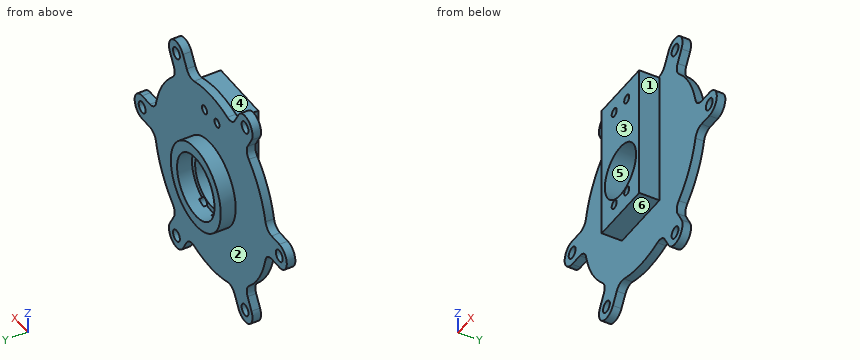
```python
from build123d import *

# Parameters (mm, degrees)
SKETCH_1_R               = 20
SKETCH_1_R_2             = 15
EXTRUDE_1_DEPTH          = 7
SKETCH_2_R               = 70
SKETCH_2_R_2             = 12.5
EXTRUDE_2_DEPTH          = 4
SKETCH_3_W               = 30
SKETCH_3_H               = 64
SKETCH_3_R               = 2
SKETCH_3_R_2             = 12.5
EXTRUDE_3_DEPTH          = 9.5
SKETCH_4_R               = 80
SKETCH_4_R_2             = 45
CUT_EXTRUDE_1_DEPTH      = 9.5
CUT_EXTRUDE_START        = -15
SKETCH_6_R               = 2
CUT_EXTRUDE_2_DEPTH      = 15
SKETCH_7_R               = 2.75
EXTRUDE_4_DEPTH          = 4
PATTERN_CIRCULAR_1_COUNT = 6
FILLET_2_R               = 5


with BuildPart() as part:
    # Эскиз1 → Бобышка-Вытянуть1 (new body)
    with BuildSketch(Plane(origin=(0, 0, 0), x_dir=(1, 0, 0), z_dir=(0, 1, 0))):
        with Locations(Location((0, 0, 0), (0, 0, 270))):
            Circle(SKETCH_1_R)
        with Locations(Location((0, 0, 0), (0, 0, 270))):
            Circle(SKETCH_1_R_2, mode=Mode.SUBTRACT)
    extrude(amount=EXTRUDE_1_DEPTH)

    # Эскиз2 → Бобышка-Вытянуть2 (add)
    with BuildSketch(Plane.XZ):
        with Locations(Location((0, 0, 0), (0, 0, 270))):
            Circle(SKETCH_2_R)
        with Locations(Location((0, 0, 0), (0, 0, 270))):
            Circle(SKETCH_2_R_2, mode=Mode.SUBTRACT)
    extrude(amount=EXTRUDE_2_DEPTH)

    # Эскиз3 → Бобышка-Вытянуть3 (add)
    with BuildSketch(Plane.XZ.offset(4)):
        with Locations((0, 10)):
            Rectangle(SKETCH_3_W, SKETCH_3_H)
        with Locations(Location((-5, 34, 0), (0, 0, 270))):
            Circle(SKETCH_3_R, mode=Mode.SUBTRACT)
        with Locations(Location((5, 34, 0), (0, 0, 270))):
            Circle(SKETCH_3_R, mode=Mode.SUBTRACT)
        with Locations(Location((-5, -14, 0), (0, 0, 270))):
            Circle(SKETCH_3_R, mode=Mode.SUBTRACT)
        with Locations(Location((5, -14, 0), (0, 0, 270))):
            Circle(SKETCH_3_R, mode=Mode.SUBTRACT)
        with Locations(Location((0, 0, 0), (0, 0, 270))):
            Circle(SKETCH_3_R_2, mode=Mode.SUBTRACT)
    extrude(amount=EXTRUDE_3_DEPTH)

    # Эскиз4 → Вырез-Вытянуть1 (cut)
    with BuildSketch(Plane(origin=(0, 0, 0), x_dir=(1, 0, 0), z_dir=(0, 1, 0))):
        Circle(SKETCH_4_R)
        with Locations(Location((0, 0, 0), (0, 0, 270))):
            Circle(SKETCH_4_R_2, mode=Mode.SUBTRACT)
    extrude(amount=-CUT_EXTRUDE_1_DEPTH, mode=Mode.SUBTRACT)

    # Эскиз6 → Вырез-Вытянуть2 (cut)
    with BuildSketch(Plane.XZ.offset(13.5).offset(CUT_EXTRUDE_START)):
        with Locations(Location((-5, 34, 0), (0, 0, 270))):
            Circle(SKETCH_6_R)
        with Locations(Location((5, 34, 0), (0, 0, 270))):
            Circle(SKETCH_6_R)
        with Locations(Location((-5, -14, 0), (0, 0, 160.346175942))):
            Circle(SKETCH_6_R)
        with Locations(Location((5, -14, 0), (0, 0, 19.653824058))):
            Circle(SKETCH_6_R)
    extrude(amount=CUT_EXTRUDE_2_DEPTH, mode=Mode.SUBTRACT)

    # Эскиз7 → Бобышка-Вытянуть4 (add)
    with BuildSketch(Plane(origin=(0, 0, 0), x_dir=(1, 0, 0), z_dir=(0, 1, 0))):
        with BuildLine():
            Line((-55, 6), (-40, 6))
            Line((-40, 6), (-40, -6))
            Line((-40, -6), (-55, -6))
            ThreePointArc((-55, -6), (-61, 0), (-55, 6))
        make_face()
        with Locations(Location((-55, 0, 0), (0, 0, 270))):
            Circle(SKETCH_7_R, mode=Mode.SUBTRACT)
    extrude_4 = extrude(amount=-EXTRUDE_4_DEPTH)

    # Круговой массив1: Бобышка-Вытянуть4 ×6 about axis
    pattern_circular_1_axis = Axis((0, 0, 0), (0, 1, 0))
    for i in range(1, PATTERN_CIRCULAR_1_COUNT):
        add(extrude_4.rotate(pattern_circular_1_axis, i * 360 / PATTERN_CIRCULAR_1_COUNT))

    # Скругление2
    fillet_2_edges = [part.edges().sort_by_distance(p)[0] for p in [
        (-17.102950698, -2, 41.623179569),
        (-27.495255544, -2, 35.623179569),
        (27.495255544, -2, 35.623179569),
        (17.102950698, -2, 41.623179569),
        (44.598206242, -2, -6),
        (44.598206242, -2, 6),
        (17.102950698, -2, -41.623179569),
        (27.495255544, -2, -35.623179569),
        (-27.495255544, -2, -35.623179569),
        (-17.102950698, -2, -41.623179569),
        (-44.598206242, -2, 6),
        (-44.598206242, -2, -6),
    ]]
    fillet(fillet_2_edges, radius=FILLET_2_R)


solid = part.part
```
Verification items for the finished model (mm, model axes). Face numbers are marked on the shaded views. A direction names the side the tool comes from. Give positions to 0.01 mm unless a question says otherwise; leave off trailing zeros. Order: outer loops, then holes, each group sorted by start corner. A loop starts at its lowest first (then second) coordinate and runs counter-clockwise, first axis right, second up. Notation, with made-up numbers: M 80.5,-39 L 132.5,-39 A29 ccw 132.5,-17 Z; hole C 47.5,-36.5 d11. An arc over 180 degrees is marked long. Return JSON: item names as keys, results as strings. Group by question number.
1) Mould release check, pull along Z, two halves, no side actions. Record for the marked faces 3, 4, 5 and 6: pulls with the +Z half, pulls with the -Z half, needs draft (parallel to the pull), parting line crosses it, or undercut.
2) Access from +Z, -Z, +X, -X, +Y, -Y to the whole of each face (thin tool, end or side, straight path). Record for the marked faces 1 and 2.
3) Section check B-B on x = -27.5. Record the cut outline in (y, z), and give its area (3 significant figures).
4) Section check C-C on y = -11.25. Record the cut outline in (x, z), and give its area (3 significant figures).
5) Scan lines: line 1 (X direction, y = -2.75, z = 0); line 2 (X direction, y = -1.5, z = -1); line 3 (Y direction, x = 43, z = 2). Record each from-to range of solid material in increasing order.
6) Section check D-D on x = 0. Record the cut outline in (y, z).
7) Section check A-A on z = 0. Record the cut outline in (x, y).
8) Go/stop test with flat-tipped pins: pin 1 Ø8 at (x, y) = (-23, 1.5) entering from +Z; pin 2 Ø10.5 at (y, z) = (-9.5, 2) entering from +X; pin 3 Ø2 at (x, y) = (51, -2.5) entering from +Z; pin 4 Ø3.5 at (x, z) = (5, 34) entering from +Y. Record where each tip stops, or that it passes through.
Answer block:
{
 "1": {"face 3": "needs draft", "face 4": "pulls with the +Z half", "face 5": "undercut", "face 6": "pulls with the -Z half"},
 "2": {"face 1": "+Z, -Z, +X, -Y", "face 2": "+Y"},
 "3": {"outline": "M -4,-53.63 L 0,-53.63 L 0,-50.38 L -4,-50.38 Z; M -4,-44.88 L 0,-44.88 L 0,44.88 L -4,44.88 Z; M -4,50.38 L 0,50.38 L 0,53.63 L -4,53.63 Z", "area": "385 mm^2"},
 "4": {"outline": "M -15,-22 L 15,-22 L 15,42 L -15,42 Z; hole C 0,0 d25; hole C -5,-14 d4; hole C -5,34 d4; hole C 5,-14 d4; hole C 5,34 d4", "area": "1,380 mm^2"},
 "5": {"line 1": "x = -61 to -57.75, -52.25 to -12.5, 12.5 to 52.25, 57.75 to 61", "line 2": "x = -60.92 to -57.56, -52.44 to -12.46, 12.46 to 52.44, 57.56 to 60.92", "line 3": "y = -4 to 0"},
 "6": {"outline": "M -13.5,-22 L -4,-22 L -4,-45 L 0,-45 L 0,-20 L 7,-20 L 7,-15 L 0,-15 L 0,-12.5 L -13.5,-12.5 Z; M -13.5,12.5 L 0,12.5 L 0,15 L 7,15 L 7,20 L 0,20 L 0,45 L -4,45 L -4,42 L -13.5,42 Z"},
 "7": {"outline": "M -61,-4 L -57.75,-4 L -57.75,0 L -61,0 Z; M -52.25,-4 L -15,-4 L -15,-13.5 L -12.5,-13.5 L -12.5,0 L -15,0 L -15,7 L -20,7 L -20,0 L -52.25,0 Z; M 12.5,-13.5 L 15,-13.5 L 15,-4 L 52.25,-4 L 52.25,0 L 20,0 L 20,7 L 15,7 L 15,0 L 12.5,0 Z; M 57.75,-4 L 61,-4 L 61,0 L 57.75,0 Z"},
 "8": {"pin 1": "stops at z = 53.58", "pin 2": "stops at x = 15", "pin 3": "stops at z = 6", "pin 4": "passes through"}
}
